The listing builds one solid part. Answer for the finished solid, in the listing's coordinates (mm). A direction names the side the tool comes from. Round coordinates to 2 decimals unless told otherwise and drop trailing zeros. Loops run counter-clockwise (first coordinate to the right, second up) from the corner with the lowest first, then second, coordinate; pieces in that order, holes last. Notation, with made-up numbers: (18.25, 74) -> (69.25, 74) arc R12 ccw to (69.25, 94) -> close; hole circle Ø11 at (-16, 59.25). An arc over 180 degrees is marked (long way). Write each question's results on one line, items separated by ' | '. Start each with the question number.
from build123d import *

# Parameters (mm, degrees)
SKETCH1_R                = 140
SKETCH1_R_2              = 96
BOSS_EXTRUDE1_DEPTH      = 225
SKETCH2_R                = 23.5
BOSS_EXTRUDE2_DEPTH      = 32
CIRPATTERN1_COUNT        = 3
MIRROR1_COPY_1_SKETCH_R  = 23.5
MIRROR1_COPY_1_DEPTH     = 32
MIRROR1_COPY_2_SKETCH_R  = 23.5
MIRROR1_COPY_2_DEPTH     = 32
BOSS_EXTRUDE3_REACH      = 491.361
BOSS_EXTRUDE3_END_RADIUS = 140
SKETCH3_R                = 100
SKETCH4_R                = 50
CUT_EXTRUDE1_DEPTH       = 25
SKETCH5_R                = 28
CUT_EXTRUDE2_DEPTH       = 470.945948606
SKETCH7_R                = 12
CUT_EXTRUDE3_DEPTH       = 15
CIRPATTERN2_COUNT        = 3


with BuildPart() as part:
    # Sketch1 → Boss-Extrude1 (new body)
    with BuildSketch(Plane(origin=(0, 0, 0), x_dir=(1, 0, 0), z_dir=(0, 1, 0))):
        with Locations(Location((0, 0, 0), (0, 0, 270))):
            Circle(SKETCH1_R)
        with Locations(Location((0, 0, 0), (0, 0, 270))):
            Circle(SKETCH1_R_2, mode=Mode.SUBTRACT)
    extrude(amount=BOSS_EXTRUDE1_DEPTH)

    # Sketch2 → Boss-Extrude2 (add)
    with BuildSketch(Plane(origin=(0, 225, 0), x_dir=(1, 0, 0), z_dir=(0, 1, 0))):
        with BuildLine():
            Line((50, 175), (50, 130.766968306))
            Line((50, 130.766968306), (-50, 130.766968306))
            Line((-50, 130.766968306), (-50, 175))
            ThreePointArc((-50, 175), (0, 225), (50, 175))
        make_face()
        with Locations(Location((0, 175, 0), (0, 0, 270))):
            Circle(SKETCH2_R, mode=Mode.SUBTRACT)
    boss_extrude2 = extrude(amount=-BOSS_EXTRUDE2_DEPTH)

    # CirPattern1: Boss-Extrude2 ×3 about axis
    cirpattern1_axis = Axis((0, 0, 0), (0, 1, 0))
    for i in range(1, CIRPATTERN1_COUNT):
        add(boss_extrude2.rotate(cirpattern1_axis, i * 360 / CIRPATTERN1_COUNT))

    # Mirror1: Boss-Extrude2 across plane
    add(boss_extrude2.mirror(Plane.ZX.offset(112.5)))

    # Mirror1 copy 1 sketch → Mirror1 copy 1 (add)
    with BuildSketch(Plane(origin=(0, 0, 0), x_dir=(-0.4999999999999998, 0, -0.8660254037844387), z_dir=(0, -1, 0))):
        with BuildLine():
            Line((50, -175), (50, -130.766968306))
            Line((50, -130.766968306), (-50, -130.766968306))
            Line((-50, -130.766968306), (-50, -175))
            ThreePointArc((-50, -175), (0, -225), (50, -175))
        make_face()
        with Locations((0, -175)):
            Circle(MIRROR1_COPY_1_SKETCH_R, mode=Mode.SUBTRACT)
    extrude(amount=-MIRROR1_COPY_1_DEPTH)

    # Mirror1 copy 2 sketch → Mirror1 copy 2 (add)
    with BuildSketch(Plane(origin=(0, 0, 0), x_dir=(-0.5000000000000004, 0, 0.8660254037844384), z_dir=(0, -1, 0))):
        with BuildLine():
            Line((50, -175), (50, -130.766968306))
            Line((50, -130.766968306), (-50, -130.766968306))
            Line((-50, -130.766968306), (-50, -175))
            ThreePointArc((-50, -175), (0, -225), (50, -175))
        make_face()
        with Locations((0, -175)):
            Circle(MIRROR1_COPY_2_SKETCH_R, mode=Mode.SUBTRACT)
    extrude(amount=-MIRROR1_COPY_2_DEPTH)

    # Boss-Extrude3: up to this cylinder (the profile starts outside it)
    boss_extrude3_end = Plane(origin=(0, 112.5, 0), z_dir=(0, -1, 0)) * Cylinder(BOSS_EXTRUDE3_END_RADIUS, 1263.722, mode=Mode.PRIVATE)
    # Sketch3 → Boss-Extrude3 (add, up to the surface)
    with BuildSketch(Plane.XY.offset(160), mode=Mode.PRIVATE) as boss_extrude3_sk1:
        with Locations((0, 112.5)):
            Circle(SKETCH3_R)
    boss_extrude3_tool1 = extrude(boss_extrude3_sk1.sketch, amount=-BOSS_EXTRUDE3_REACH, mode=Mode.PRIVATE) - boss_extrude3_end
    add(boss_extrude3_tool1.solids().sort_by_distance((0, 112.5, 160))[0])

    # Sketch4 → Cut-Extrude1 (cut)
    with BuildSketch(Plane.XY.offset(160)):
        with Locations((3.778615411, 116.042451948)):
            Circle(SKETCH4_R)
    extrude(amount=-CUT_EXTRUDE1_DEPTH, mode=Mode.SUBTRACT)

    # Sketch5 → Cut-Extrude2 (cut, through all)
    with BuildSketch(Plane.XY.offset(135)):
        with Locations((3.778615411, 116.042451948)):
            Circle(SKETCH5_R)
    extrude(amount=-CUT_EXTRUDE2_DEPTH, mode=Mode.SUBTRACT)

    # Sketch7 → Cut-Extrude3 (cut)
    with BuildSketch(Plane.XY.offset(160)):
        with Locations((0, 191.042451948)):
            Circle(SKETCH7_R)
    cut_extrude3 = extrude(amount=-CUT_EXTRUDE3_DEPTH, mode=Mode.SUBTRACT)

    # CirPattern2: Cut-Extrude3 ×3 about axis
    cirpattern2_axis = Axis((0, 112.5, 0), (0, 0, 1))
    for i in range(1, CIRPATTERN2_COUNT):
        add(cut_extrude3.rotate(cirpattern2_axis, i * 360 / CIRPATTERN2_COUNT), mode=Mode.SUBTRACT)


solid = part.part
Item 1: The part is cut by section B-B, the plane y = 106.5. Give the vertices of the cut face in (x, z), plus the area to 3 significant figures.
Item 2: The part is cut by section A-A, the plane z = 0. Give the vertices of the cut face in (x, y), plus the area to 3 significant figures.
Item 3: Straight lines are drawn through the part: L1, parallel to Z at x = -15.5, y = 19; L2, parallel to Y at x = 136.5, z = 34; L3, parallel to Z at x = -14.5, y = 82. For each, find the intervals that lie inside material, in ascending order. Write a range as [from, to].
Item 4: Each of these flat-tipped pins is pushed along its axis until it touches: pin 1 Ø14.5 at (x, y) = (68.02, 73.23) entering from +Z; pin 2 Ø16 at (y, z) = (20, -142) entering from +X; pin 3 Ø8 at (y, z) = (110, -9) entering from -X. Where does it stop, or does it pass through?
Item 5: The part is cut by section D-D, the plane y = 26. Give the vertices of the cut face in (x, z), plus the area to 3 significant figures.
Item 6: The part is cut by section C-C, the plane x = 161. Give the vertices of the cut face in (y, z).
Item 7: Determine the mould class of faces 1 (the flat face through (-78, 225, 60)), 2 (the cylindrical face through (30.486, 124.453, 113.105)), 3 (the cylindrical face through (1.033, 209.224, -198.477)) for opening direction Y: +Y half, -Y half, draft (parallel to the pull), parting line (faces both ways), or undercut.
Item 8: For faces 4 (the flat face through (-50, 16, -153)), 5 (the cylindrical face through (-1.56, 202.94, 152.6)), 6 (the flat face through (-107.133, 15.776, 119.588)), 7 (the flat face through (-173, 193, 99)), 8 (the flat face through (166, 32, 108)), determine the directions among +Z, -Z, +X, -X, +Y, -Y from which every point of the face is accessible in a straight line to the end or side of a thin tool.
Report:
1) outline: (-99.82, 98.16) arc R140 ccw to (-22.55, -138.17) -> (-22.55, -93.32) arc R96 cw to (-22.55, 93.32) -> (-22.55, 135) -> (-45.3, 135) -> (-45.3, 160) -> (-99.82, 160) -> close; (30.1, -136.73) arc R140 ccw to (99.82, 98.16) -> (99.82, 160) -> (52.86, 160) -> (52.86, 135) -> (30.1, 135) -> (30.1, 91.16) arc R96 cw to (30.1, -91.16) -> close | area: 32,300 mm2
2) outline: (-140, 0) -> (-96, 0) -> (-96, 225) -> (-140, 225) -> close; (96, 0) -> (140, 0) -> (140, 225) -> (96, 225) -> close | area: 19,800 mm2
3) L1: z = [-222.54, -192.66], [-157.34, -94.74], [94.74, 160] | L2: y = [0, 32], [193, 225] | L3: z = [-139.25, -94.9], [94.9, 135]
4) pin 1: stops at z = 145 | pin 2: stops at x = 50 | pin 3: stops at x = -139.91
5) outline: (-176.55, 44.2) -> (-138.25, 22.08) arc R140 ccw to (-50, -130.77) -> (-50, -175) arc R50 ccw to (50, -175) -> (50, -130.77) arc R140 ccw to (138.25, 22.08) -> (176.55, 44.2) arc R50 ccw to (126.55, 130.8) -> (88.25, 108.68) arc R140 ccw to (50.18, 130.7) -> (50.18, 160) -> (-50.18, 160) -> (-50.18, 130.7) arc R140 ccw to (-88.25, 108.68) -> (-126.55, 130.8) arc R50 ccw to start; hole circle Ø47 at (-151.55, 87.5); hole circle Ø192 at (0, 0); hole circle Ø47 at (0, -175); hole circle Ø47 at (151.55, 87.5) | area: 52,900 mm2
6) outline: (0, 35.22) -> (32, 35.22) -> (32, 65.98) -> (0, 65.98) -> close; (0, 109.02) -> (32, 109.02) -> (32, 136.6) -> (0, 136.6) -> close; (193, 35.22) -> (225, 35.22) -> (225, 65.98) -> (193, 65.98) -> close; (193, 109.02) -> (225, 109.02) -> (225, 136.6) -> (193, 136.6) -> close
7) face 1: +Y half | face 2: undercut | face 3: draft
8) face 4: -Z, -X, +Y, -Y | face 5: +Z | face 6: +Z, -Y | face 7: +Z, -X | face 8: +Z, +X
